Part model, mm, in its own coordinate system. A direction names the side the tool comes from. Round coordinates to 2 decimals unless told otherwise and drop trailing zeros. Order: outer loops, then holes, each group sorted by start corner. A loop starts at its lowest first (then second) coordinate and runs counter-clockwise, first axis right, second up. Notation, with made-up numbers: (76.5, 14.5) - (99.5, 14.5) arc R7 cw to (99.5, 21.5) - close; hole circle Ø5 at (-38, 64). An arc over 180 degrees is marked (long way). Answer as a JSON object with one key per item and string values.
```python
from build123d import *

# Parameters (mm, degrees)
SKETCH1_R            = 70
SKETCH1_R_2          = 45
BOSS_EXTRUDE1_DEPTH  = 4
SKETCH3_R            = 60
SKETCH3_R_2          = 45
BOSS_EXTRUDE4_DEPTH  = 32
SKETCH6_W            = 16
SKETCH6_H            = 10
SKETCH6_W_2          = 34
BOSS_EXTRUDE5_DEPTH  = 12.5
SKETCH10_W           = 15
SKETCH10_H           = 22
BOSS_EXTRUDE6_DEPTH  = 12.5
SKETCH11_W           = 34
SKETCH11_H           = 4
BOSS_EXTRUDE7_DEPTH  = 30
SKETCH12_W           = 17.229041164
SKETCH12_H           = 10
CUT_EXTRUDE3_DEPTH   = 12.5
CUT_EXTRUDE4_DEPTH   = 12.5
CUT_EXTRUDE5_DEPTH   = 12.5
SKETCH20_W           = 10
SKETCH20_H           = 25
CUT_EXTRUDE11_DEPTH  = 4
SKETCH21_R           = 45
SKETCH21_R_2         = 32.5
BOSS_EXTRUDE8_DEPTH  = 15
SKETCH22_W           = 17.163263372
SKETCH22_H           = 25
CUT_EXTRUDE12_DEPTH  = 5
SKETCH25_R           = 63
SKETCH25_R_2         = 60
BOSS_EXTRUDE9_DEPTH  = 50
SKETCH26_R           = 80
SKETCH26_R_2         = 70
BOSS_EXTRUDE10_DEPTH = 4
SKETCH29_R           = 3
CUT_EXTRUDE14_DEPTH  = 5
SKETCH30_R           = 80
SKETCH30_R_2         = 3
BOSS_EXTRUDE11_DEPTH = 10
SKETCH16_R           = 6
CUT_EXTRUDE10_DEPTH  = 100
SKETCH31_W           = 42
SKETCH31_H           = 25
CUT_EXTRUDE15_DEPTH  = 1
SKETCH33_R           = 81.797304038
SKETCH33_R_2         = 27.899813831
CUT_EXTRUDE17_DEPTH  = 37.5
SKETCH34_R           = 1.5
CUT_EXTRUDE18_DEPTH  = 10


with BuildPart() as part:
    # Sketch1 → Boss-Extrude1 (new body)
    with BuildSketch(Plane.XY):
        Circle(SKETCH1_R)
        Circle(SKETCH1_R_2, mode=Mode.SUBTRACT)
    extrude(amount=BOSS_EXTRUDE1_DEPTH)

    # Sketch3 → Boss-Extrude4 (add)
    with BuildSketch(Plane.XY):
        Circle(SKETCH3_R)
        Circle(SKETCH3_R_2, mode=Mode.SUBTRACT)
    extrude(amount=BOSS_EXTRUDE4_DEPTH)

    # Sketch6 → Boss-Extrude5 (add, symmetric)
    with BuildSketch(Plane(origin=(0, 0, 0), x_dir=(1, 0, 0), z_dir=(0, 1, 0))):
        with Locations((37, -27)):
            Rectangle(SKETCH6_W, SKETCH6_H)
        with Locations((-28, -27)):
            Rectangle(SKETCH6_W_2, SKETCH6_H)
    extrude(amount=BOSS_EXTRUDE5_DEPTH, both=True)

    # Sketch10 → Boss-Extrude6 (add, symmetric)
    with BuildSketch(Plane(origin=(0, 0, 0), x_dir=(1, 0, 0), z_dir=(0, 1, 0))):
        with Locations((-18.5, -11)):
            Rectangle(SKETCH10_W, SKETCH10_H)
    extrude(amount=BOSS_EXTRUDE6_DEPTH, both=True)

    # Sketch11 → Boss-Extrude7 (add, symmetric)
    with BuildSketch(Plane(origin=(0, 0, 0), x_dir=(1, 0, 0), z_dir=(0, 1, 0))):
        with Locations((-28, -2)):
            Rectangle(SKETCH11_W, SKETCH11_H)
    extrude(amount=BOSS_EXTRUDE7_DEPTH, both=True)

    # Sketch12 → Cut-Extrude3 (cut, symmetric)
    with BuildSketch(Plane(origin=(0, 0, 0), x_dir=(1, 0, 0), z_dir=(0, 1, 0))):
        with Locations((-34.614520582, -27)):
            Rectangle(SKETCH12_W, SKETCH12_H)
    extrude(amount=CUT_EXTRUDE3_DEPTH, both=True, mode=Mode.SUBTRACT)

    # Sketch13 → Cut-Extrude4 (cut, symmetric)
    with BuildSketch(Plane.XY):
        Polygon((-33.541019662, 30), (-11, 12.5), (-11, 30), align=None)
    extrude(amount=CUT_EXTRUDE4_DEPTH, both=True, mode=Mode.SUBTRACT)

    # Sketch14 → Cut-Extrude5 (cut, symmetric)
    with BuildSketch(Plane.XY):
        Polygon((-33.541019662, -30), (-11, -12.5), (-11, -30), align=None)
    extrude(amount=CUT_EXTRUDE5_DEPTH, both=True, mode=Mode.SUBTRACT)

    # Sketch20 → Cut-Extrude11 (cut)
    with BuildSketch(Plane.XY.offset(32)):
        with Locations((-16, 0)):
            Rectangle(SKETCH20_W, SKETCH20_H)
        with Locations((34, 0)):
            Rectangle(SKETCH20_W, SKETCH20_H)
    extrude(amount=-CUT_EXTRUDE11_DEPTH, mode=Mode.SUBTRACT)

    # Sketch21 → Boss-Extrude8 (add)
    with BuildSketch(Plane.XY.offset(32)):
        Circle(SKETCH21_R)
        Circle(SKETCH21_R_2, mode=Mode.SUBTRACT)
    extrude(amount=-BOSS_EXTRUDE8_DEPTH)

    # Sketch22 → Cut-Extrude12 (cut)
    with BuildSketch(Plane.XY.offset(32)):
        with Locations((34.647409478, 0)):
            Rectangle(SKETCH22_W, SKETCH22_H)
    extrude(amount=-CUT_EXTRUDE12_DEPTH, mode=Mode.SUBTRACT)

    # Sketch25 → Boss-Extrude9 (add)
    with BuildSketch(Plane.XY.offset(4)):
        Circle(SKETCH25_R)
        Circle(SKETCH25_R_2, mode=Mode.SUBTRACT)
    extrude(amount=BOSS_EXTRUDE9_DEPTH)

    # Sketch26 → Boss-Extrude10 (add)
    with BuildSketch(Plane(origin=(0, 0, 0), x_dir=(-1, 0, 0), z_dir=(0, 0, -1))):
        Circle(SKETCH26_R)
        Circle(SKETCH26_R_2, mode=Mode.SUBTRACT)
    extrude(amount=-BOSS_EXTRUDE10_DEPTH)

    # Sketch29 → Cut-Extrude14 (cut)
    with BuildSketch(Plane.XY.offset(4)):
        with Locations((0, 70)):
            Circle(SKETCH29_R)
        with Locations((60.621778265, 35)):
            Circle(SKETCH29_R)
        with Locations((60.621778265, -35)):
            Circle(SKETCH29_R)
        with Locations((0, -70)):
            Circle(SKETCH29_R)
        with Locations((-60.621778265, -35)):
            Circle(SKETCH29_R)
        with Locations((-60.621778265, 35)):
            Circle(SKETCH29_R)
    extrude(amount=-CUT_EXTRUDE14_DEPTH, mode=Mode.SUBTRACT)

    # Sketch30 → Boss-Extrude11 (add)
    with BuildSketch(Plane(origin=(0, 0, 0), x_dir=(-1, 0, 0), z_dir=(0, 0, -1))):
        Circle(SKETCH30_R)
        with Locations((-60.621778265, 35)):
            Circle(SKETCH30_R_2, mode=Mode.SUBTRACT)
        with Locations((-60.621778265, -35)):
            Circle(SKETCH30_R_2, mode=Mode.SUBTRACT)
        with Locations((0, -70)):
            Circle(SKETCH30_R_2, mode=Mode.SUBTRACT)
        with Locations((60.621778265, -35)):
            Circle(SKETCH30_R_2, mode=Mode.SUBTRACT)
        with Locations((60.621778265, 35)):
            Circle(SKETCH30_R_2, mode=Mode.SUBTRACT)
        with Locations((0, 70)):
            Circle(SKETCH30_R_2, mode=Mode.SUBTRACT)
        with BuildLine():
            Line((11, -12.5), (33.541019662, -30))
            ThreePointArc((33.541019662, -30), (-45, 0), (33.541019662, 30))
            Line((33.541019662, 30), (11, 12.5))
            Line((11, 12.5), (11, -12.5))
        make_face(mode=Mode.SUBTRACT)
    extrude(amount=BOSS_EXTRUDE11_DEPTH)

    # Sketch16 → Cut-Extrude10 (cut)
    with BuildSketch(Plane(origin=(-11, 0, 0), x_dir=(0, 0, -1), z_dir=(1, 0, 0))):
        with Locations((-10, 0)):
            Circle(SKETCH16_R)
    extrude(amount=-CUT_EXTRUDE10_DEPTH, mode=Mode.SUBTRACT)

    # Sketch31 → Cut-Extrude15 (cut)
    with BuildSketch(Plane.XY.offset(28)):
        Rectangle(SKETCH31_W, SKETCH31_H)
    extrude(amount=-CUT_EXTRUDE15_DEPTH, mode=Mode.SUBTRACT)

    # Sketch33 → Cut-Extrude17 (cut)
    with BuildSketch(Plane.XY.offset(54)):
        Circle(SKETCH33_R)
        Circle(SKETCH33_R_2, mode=Mode.SUBTRACT)
    extrude(amount=-CUT_EXTRUDE17_DEPTH, mode=Mode.SUBTRACT)

    # Sketch34 → Cut-Extrude18 (cut)
    with BuildSketch(Plane.XY.offset(27)):
        with Locations((-14, 6)):
            Circle(SKETCH34_R)
        with Locations((-14, -6)):
            Circle(SKETCH34_R)
    extrude(amount=-CUT_EXTRUDE18_DEPTH, mode=Mode.SUBTRACT)


solid = part.part
```
Item 1: Cut at D-D (y = 15). Write the cut outline in (x, z).
Taken from the geometry:
{"outline": "(-78.58, -10) - (-14.22, -10) - (-14.22, 4) - (-42.43, 4) - (-42.43, 16.5) - (-61.19, 16.5) - (-61.19, 4) - (-78.58, 4) - close; (42.43, -10) - (78.58, -10) - (78.58, 4) - (61.19, 4) - (61.19, 16.5) - (42.43, 16.5) - close"}
Item 2: Cut at A-A (x = 0). Write the cut outline in (y, z).
Taken from the geometry:
{"outline": "(-80, -10) - (-73, -10) - (-73, 4) - (-80, 4) - close; (-67, -10) - (-45, -10) - (-45, 16.5) - (-63, 16.5) - (-63, 4) - (-67, 4) - close; (45, -10) - (67, -10) - (67, 4) - (63, 4) - (63, 16.5) - (45, 16.5) - close; (73, -10) - (80, -10) - (80, 4) - (73, 4) - close"}
Item 3: Two-plate mould, pull along Y, no slides. Class faces 4 (the cylindrical face through (-18.395, 1.802, 4.277)), 5 (the flat face through (-16, 0, 27)), 6 (the cylindrical face through (60.1, 18.9, 10.2)): pulls with the +Y half, pulls with the -Y half, needs draft (parallel to the pull), parting line crosses it, or undercut.
Taken from the geometry:
{"face 4": "undercut", "face 5": "needs draft", "face 6": "parting line crosses it"}
Item 4: Tool access for faces 1 (the cylindrical face through (-53.67, 1.802, 4.277)), 2 (the flat face through (-19, -12.5, 15)), 3 (the flat face through (-24, 0, 32)): list every direction of +Z, -Z, +X, -X, +Y, -Y with a clear straight run to the whole face (end or side of a thin tool).
Taken from the geometry:
{"face 1": "-X", "face 2": "+Z", "face 3": "+Z, +X, -X, +Y, -Y"}
Item 5: Probe L1, parallel to Y at x = 0, z = -5; L2, parallel to X at y = -35, z = -7; L3, parallel to Z at x = -35, y = 9.5. List the from-to ranges inside material, lowest first. Write a range as from..to.
Taken from the geometry:
{"L1": "-80..-73, -67..-45, 45..67, 73..80", "L2": "-71.94..-63.62, -57.62..-28.28, 28.28..57.62, 63.62..71.94", "L3": "-10..4"}
Item 6: Cut at C-C (y = 35). Write the cut outline in (x, z), plus the area to 3 significant figures.
Taken from the geometry:
{"outline": "(-71.94, -10) - (-63.62, -10) - (-63.62, 4) - (-71.94, 4) - close; (-57.62, -10) - (-28.28, -10) - (-28.28, 16.5) - (-52.38, 16.5) - (-52.38, 4) - (-57.62, 4) - close; (28.28, -10) - (57.62, -10) - (57.62, 4) - (52.38, 4) - (52.38, 16.5) - (28.28, 16.5) - close; (63.62, -10) - (71.94, -10) - (71.94, 4) - (63.62, 4) - close", "area": "1,660 mm2"}
Item 7: Drop flat-ended pins along their axis: P1, Ø8, axis at x = 48, y = 38, coming from the +Z side; P2, Ø5, axis at x = -17, y = 2, coming from the +Z side; P3, Ø6, axis at y = -19, z = 2, coming from the +X side; P4, Ø5, axis at x = 0, y = 70, coming from the -Z side. Give the stop position or say it passes through.
Taken from the geometry:
{"P1": "z = 16.5", "P2": "z = 27", "P3": "x = 78.38", "P4": "through"}
Item 8: Cut at B-B (z = 10). Write the cut outline in (x, y).
Taken from the geometry:
{"outline": "(-62.71, -6) arc R63 ccw (long way) to (-62.71, 6) - (-44.6, 6) arc R45 cw (long way) to (-44.6, -6) - close; (-26, -12.5) - (-11, -12.5) - (-11, -6) - (-26, -6) - close; (-26, 6) - (-11, 6) - (-11, 12.5) - (-26, 12.5) - close"}
